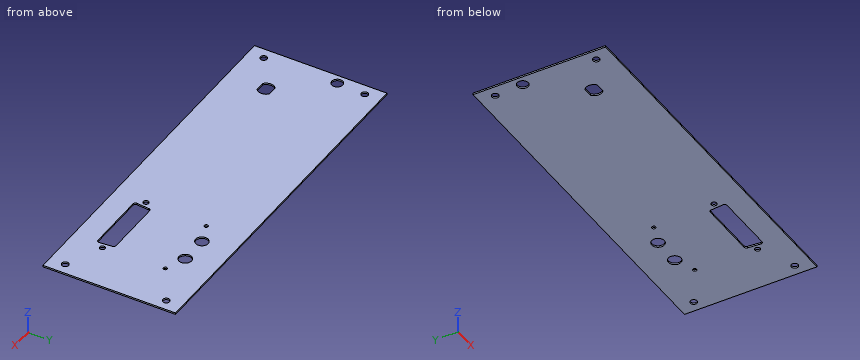
```python
from build123d import *

# Parameters (mm, degrees)
SKETCH_1_W          = 228
SKETCH_1_H          = 84
SKETCH_1_R          = 2.15
EXTRUDE_1_DEPTH     = 1
SKETCH_3_R          = 1.7
SKETCH_3_R_2        = 1.2
SKETCH_3_R_3        = 4
CUT_EXTRUDE_1_DEPTH = 10
SKETCH_4_R          = 3.5
CUT_EXTRUDE_2_DEPTH = 1


with BuildPart() as part:
    # Эскиз1 → Вытянуть1 (new body)
    with BuildSketch(Plane.XY):
        Rectangle(SKETCH_1_W, SKETCH_1_H)
        with Locations((107, 32)):
            Circle(SKETCH_1_R, mode=Mode.SUBTRACT)
        with Locations(Location((-107, 32, 0), (0, 0, 180))):
            Circle(SKETCH_1_R, mode=Mode.SUBTRACT)
        with Locations((-107, -32)):
            Circle(SKETCH_1_R, mode=Mode.SUBTRACT)
        with Locations(Location((107, -32, 0), (0, 0, 180))):
            Circle(SKETCH_1_R, mode=Mode.SUBTRACT)
    extrude(amount=EXTRUDE_1_DEPTH)

    # Эскиз3 → Вырез-Вытянуть1 (cut)
    with BuildSketch(Plane.XY.offset(1)):
        with Locations((37, -22)):
            Circle(SKETCH_3_R)
        with Locations((84, -22)):
            Circle(SKETCH_3_R)
        with Locations((38.5, 17)):
            Circle(SKETCH_3_R_2)
        with Locations((82.5, 17)):
            Circle(SKETCH_3_R_2)
        with Locations((51.5, 22)):
            Circle(SKETCH_3_R_3)
        with Locations((69.5, 22)):
            Circle(SKETCH_3_R_3)
        with BuildLine():
            Line((40.14870942, -25.864196381), (40.875982147, -17.864196381))
            ThreePointArc((40.875982147, -17.864196381), (41.358314525, -16.892366164), (42.369821957, -16.5))
            Line((42.369821957, -16.5), (78.630178043, -16.5))
            ThreePointArc((78.630178043, -16.5), (79.641685475, -16.892366164), (80.124017853, -17.864196381))
            Line((80.124017853, -17.864196381), (80.85129058, -25.864196381))
            ThreePointArc((80.85129058, -25.864196381), (80.465084606, -27.011507432), (79.35745077, -27.5))
            Line((79.35745077, -27.5), (41.64254923, -27.5))
            ThreePointArc((41.64254923, -27.5), (40.534915394, -27.011507432), (40.14870942, -25.864196381))
        make_face()
    extrude(amount=-CUT_EXTRUDE_1_DEPTH, mode=Mode.SUBTRACT)

    # Эскиз4 → Вырез-Вытянуть2 (cut)
    with BuildSketch(Plane.XY.offset(1)):
        with Locations((-108, 14)):
            Circle(SKETCH_4_R)
        with BuildLine():
            Line((-87, -13), (-81, -13))
            ThreePointArc((-81, -13), (-79, -17), (-81, -21))
            Line((-81, -21), (-87, -21))
            ThreePointArc((-87, -21), (-89, -17), (-87, -13))
        make_face()
    extrude(amount=-CUT_EXTRUDE_2_DEPTH, mode=Mode.SUBTRACT)


solid = part.part
```
Could you check a few things on this model? Use its own coordinates, in mm. Coordinates: 2 decimals unless noted, no trailing zeros. Write each loop counter-clockwise with the first axis right and the second up, starting at its lowest first coordinate (ties: lowest second). Pieces come first, ordered by that corner, then holes. Notation, with made-up numbers: (-35.75, 36.25) - (-29.75, 36.25) arc R14 cw to (-29.75, 50.25) - close; hole circle Ø9 at (-35, 81). An arc over 180 degrees is marked (long way). Use a Markdown table: item, result.
Q1. Imagine slicing it at C-C (x = 69.5). List the corners of the cut face in (y, z) for me.
Geometry check:
| item | result |
|---|---|
| outline | (-42, 0) - (-27.5, 0) - (-27.5, 1) - (-42, 1) - close; (-16.5, 0) - (18, 0) - (18, 1) - (-16.5, 1) - close; (26, 0) - (42, 0) - (42, 1) - (26, 1) - close |
Q2. Imagine slicing it at A-A (y = 32). List the corners of the cut face in (x, z) for me.
Geometry check:
| item | result |
|---|---|
| outline | (-114, 0) - (-109.15, 0) - (-109.15, 1) - (-114, 1) - close; (-104.85, 0) - (104.85, 0) - (104.85, 1) - (-104.85, 1) - close; (109.15, 0) - (114, 0) - (114, 1) - (109.15, 1) - close |
Q3. Imagine slicing it at B-B (z = 0.7). Count the separate pieces of the cut face and the enclosed holes in it, and give its area (3 significant figures).
Geometry check:
| item | result |
|---|---|
| separate pieces | 1 |
| enclosed holes | 13 |
| area | 18,400 mm2 |
Q4. Please list where these lines run through material, in increasing order: L1, parallel to Y at x = 107, z = 0.4; L2, parallel to Y at x = 84, z = 0.6; L3, parallel to X at y = -18, z = 0.85.
Geometry check:
| item | result |
|---|---|
| L1 | y = -42 to -34.15, -29.85 to 29.85, 34.15 to 42 |
| L2 | y = -42 to -23.7, -20.3 to 42 |
| L3 | x = -114 to -88.9, -79.1 to 40.86, 80.14 to 114 |
Q5. Imagine slicing it at D-D (x = -107). List the corners of the cut face in (y, z) for me.
Geometry check:
| item | result |
|---|---|
| outline | (-42, 0) - (-34.15, 0) - (-34.15, 1) - (-42, 1) - close; (-29.85, 0) - (10.65, 0) - (10.65, 1) - (-29.85, 1) - close; (17.35, 0) - (29.85, 0) - (29.85, 1) - (17.35, 1) - close; (34.15, 0) - (42, 0) - (42, 1) - (34.15, 1) - close |
